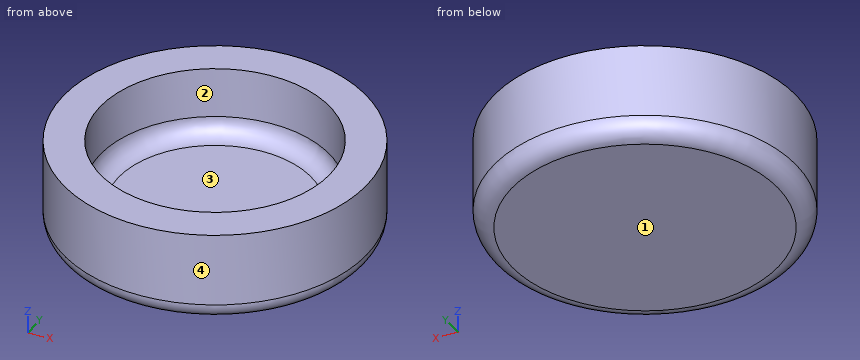
from build123d import *

# Parameters (mm, degrees)
F0_R     = 8.25
F1_DEPTH = 5
F2_R     = 6.25
F3_DEPTH = 3.75
F4_R     = 1


with BuildPart() as f1:
    # F0 (on Top) → F1 (new body)
    with BuildSketch(Plane.XY):
        Circle(F0_R)
    extrude(amount=F1_DEPTH)

    # F2 (on face) → F3 (cut)
    with BuildSketch(Plane.XY.offset(5)):
        Circle(F2_R)
    extrude(amount=-F3_DEPTH, mode=Mode.SUBTRACT)

    # F4
    f4_edges = [f1.edges().sort_by_distance(p)[0] for p in [
        (-8.25, 0, 0),
        (-6.25, 0, 1.25),
    ]]
    fillet(f4_edges, radius=F4_R)


solid = f1.part
Part model, mm, in its own coordinate system. Face numbers are marked on the shaded views. Round coordinates to 2 decimals unless told otherwise and drop trailing zeros. Write each loop counter-clockwise with the first axis right and the second up, starting at its lowest first coordinate (ties: lowest second). Pieces come first, ordered by that corner, then holes. Notation, with made-up numbers: M 31,-38.5 L 71,-38.5 A18 cw 71,-23.5 Z; hole C -5,26.5 d1. An arc over 180 degrees is marked long. Return JSON: item names as keys, results as strings. Group by question number.
(1) Saw through at C-C on z = 3.35. Write the cut outline in (x, y).
(2) Two-plate mould, pull along Y, no slides. Class the marked faces 1, 2, 3 and 4: +Y half, -Y half, draft (parallel to the pull), parting line (faces both ways), or undercut.
(3) Drill centre lines: probe 1 along Y at (x, z) = (0, 3.85); probe 2 along Z at (x, y) = (-0.25, 2.25); probe 3 along Y at (x, z) = (-1.75, 3.45). Where is each one in solid material? Low to high.
(4) Saw through at D-D on z = 0.7. Write the cut outline in (x, y), then the cut area to 3 significant figures.
(5) Saw through at A-A on y = 0. Write the cut outline in (x, z).
(6) Pin check, flat tips, straight feed: pin 1 Ø2 at (x, z) = (-2.5, 2) entering from -Y; pin 2 Ø1 at (y, z) = (-5, 3.5) entering from -X; pin 3 Ø3 at (x, y) = (0.5, -1) entering from +Z. Stop position of each tip, or through.
Returned:
{
 "1": {"outline": "C 0,0 d16.5; hole C 0,0 d12.5"},
 "2": {"face 1": "draft", "face 2": "undercut", "face 3": "undercut", "face 4": "parting line"},
 "3": {"probe 1": "-8.25 to -6.25, 6.25 to 8.25", "probe 2": "0 to 1.25", "probe 3": "-8.06 to -6, 6 to 8.06"},
 "4": {"outline": "C 0,0 d16.41", "area": "211 mm²"},
 "5": {"outline": "M -8.25,1 A1 ccw -7.25,0 L 7.25,0 A1 ccw 8.25,1 L 8.25,5 L 6.25,5 L 6.25,2.25 A1 cw 5.25,1.25 L -5.25,1.25 A1 cw -6.25,2.25 L -6.25,5 L -8.25,5 Z"},
 "6": {"pin 1": "y = -8.11", "pin 2": "x = -6.91", "pin 3": "z = 1.25"}
}
